```python
from build123d import *

# Parameters (mm, degrees)
BASE_FLANGE1_DEPTH = 631.825
SKETCH2_W          = 25.4
SKETCH2_H          = 6.35
CUT_EXTRUDE1_DEPTH = 50.8
SKETCH3_R          = 3.429
CUT_EXTRUDE2_DEPTH = 3.175
FILLET1_R          = 3.175
SKETCH4_R          = 7.9375
CUT_EXTRUDE3_DEPTH = 3.175


# Sheet-metal steps are written as plain solids
with BuildPart() as part:
    # Sketch1 → Base-Flange1 (new body)
    with BuildSketch(Plane(origin=(0, 0, 0), x_dir=(0, 0, -1), z_dir=(1, 0, 0))):
        with BuildLine():
            Line((31.75, 50.8), (6.35, 50.8))
            ThreePointArc((6.35, 50.8), (1.859871939, 48.940128061), (0, 44.45))
            Line((0, 44.45), (0, 6.35))
            ThreePointArc((0, 6.35), (1.859871939, 1.859871939), (6.35, 0))
            Line((6.35, 0), (31.75, 0))
            Line((31.75, 0), (31.75, 3.175))
            Line((31.75, 3.175), (6.35, 3.175))
            ThreePointArc((6.35, 3.175), (4.10493597, 4.10493597), (3.175, 6.35))
            Line((3.175, 6.35), (3.175, 44.45))
            ThreePointArc((3.175, 44.45), (4.10493597, 46.69506403), (6.35, 47.625))
            Line((6.35, 47.625), (31.75, 47.625))
            Line((31.75, 47.625), (31.75, 50.8))
        make_face()
    extrude(amount=BASE_FLANGE1_DEPTH)

    # Sketch2 → Cut-Extrude1 (cut)
    with BuildSketch(Plane(origin=(0, 50.8, 0), x_dir=(1, 0, 0), z_dir=(0, 1, 0))):
        with Locations((12.7, 28.575)):
            Rectangle(SKETCH2_W, SKETCH2_H)
        with Locations((619.125, 28.575)):
            Rectangle(SKETCH2_W, SKETCH2_H)
    extrude(amount=-CUT_EXTRUDE1_DEPTH, mode=Mode.SUBTRACT)

    # Sketch3 → Cut-Extrude2 (cut)
    with BuildSketch(Plane.XY):
        with Locations((22.225, 19.05)):
            Circle(SKETCH3_R)
        with Locations((22.225, 38.1)):
            Circle(SKETCH3_R)
        with Locations((622.3, 38.1)):
            Circle(SKETCH3_R)
        with BuildLine():
            Line((618.871, 22.225), (618.871, 19.05))
            ThreePointArc((618.871, 19.05), (622.3, 15.621), (625.729, 19.05))
            Line((625.729, 19.05), (625.729, 22.225))
            ThreePointArc((625.729, 22.225), (622.3, 25.654), (618.871, 22.225))
        make_face()
    extrude(amount=-CUT_EXTRUDE2_DEPTH, mode=Mode.SUBTRACT)

    # Fillet1
    fillet1_edges = [part.edges().sort_by_distance(p)[0] for p in [
        (0, 49.2125, -25.4),
        (25.4, 49.2125, -31.75),
        (0, 1.5875, -25.4),
        (25.4, 1.5875, -31.75),
        (606.425, 1.5875, -31.75),
        (606.425, 49.2125, -31.75),
        (631.825, 1.5875, -25.4),
        (631.825, 49.2125, -25.4),
        (606.425, 1.5875, -25.4),
        (606.425, 49.2125, -25.4),
        (25.4, 1.5875, -25.4),
        (25.4, 49.2125, -25.4),
    ]]
    fillet(fillet1_edges, radius=FILLET1_R - 0.0001)  # a hair under: the kernel refuses the full size

    # Sketch4 → Cut-Extrude3 (cut)
    with BuildSketch(Plane.XZ):
        with Locations(Location((41.275, -20.6375, 0), (0, 0, 270))):
            Circle(SKETCH4_R)
    extrude(amount=-CUT_EXTRUDE3_DEPTH, mode=Mode.SUBTRACT)


solid = part.part
```
The listing builds one solid part. Answer for the finished solid, in the listing's coordinates (mm). A direction names the side the tool comes from. Give positions to 0.01 mm unless a question says otherwise; leave off trailing zeros. Write each loop counter-clockwise with the first axis right and the second up, starting at its lowest first coordinate (ties: lowest second). Pieces come first, ordered by that corner, then holes. Notation, with made-up numbers: (-40, 9.5) -> (16, 9.5) arc R29 ccw to (16, 41.5) -> close; hole circle Ø7 at (35.25, 84). An arc over 180 degrees is marked (long way). Write item = value, one per line. Start each with the question number.
1) The part is cut by section A-A, the plane x = 372. Determine the outline of the cut face in (y, z) (3 decimals), and give its area (3 significant figures).
2) Which of the six approach directions +Z, -Z, +X, -X, +Y, -Y give full straight-line access (tool end or side, diameter ignored) to faces 5 (the face through (311, 3.175, -19)), 6 (the face through (311, 0, -19))?
3) Determine the mould class of faces 1 (the face through (631.825, 26, -3)), 2 (the face through (49.145, 1.565, -19.604)), 3 (the face through (311, 26, 0)), 4 (the face through (0, 26, -3)) for opening direction X: +X half, -X half, draft (parallel to the pull), parting line (faces both ways), or undercut.
4) Each of these flat-tipped pins is pushed along its axis until it touches: pin 1 (1.5 mm diameter, centred on x = 252.5, y = 45.5, fed in from +Z); pin 2 (1.6 mm diameter, centred on x = 616, y = 1.5, fed in from -Z); pin 3 (19 mm diameter, centred on x = 357.5, y = 30, fed in from -Z) (3 decimals). Where does it stop, or does it pass through?
5) Straight lines are drawn through the part: line 1 along X through (y, z) = (38, -2) (3 decimals); line 2 along Y through (x, z) = (86.5, -21) (3 decimals); line 3 along Z through (x, y) = (301, 27.5) (3 decimals). For each, find the intervals that lie inside material, in ascending order.
Solutions:
q1.outline = (0, -31.75) -> (3.175, -31.75) -> (3.175, -6.35) arc R3.175 cw to (6.35, -3.175) -> (44.45, -3.175) arc R3.175 cw to (47.625, -6.35) -> (47.625, -31.75) -> (50.8, -31.75) -> (50.8, -6.35) arc R6.35 ccw to (44.45, 0) -> (6.35, 0) arc R6.35 ccw to (0, -6.35) -> close
q1.area = 330 mm²
q2.face_5 = -Z, +X, -X
q2.face_6 = +Z, -Z, +X, -X, -Y
q3.face_1 = +X half
q3.face_2 = undercut
q3.face_3 = draft
q3.face_4 = -X half
q4.pin_1 = -0.01
q4.pin_2 = -25.4
q4.pin_3 = -3.175
q5.line_1 = 0 to 18.797, 25.653 to 618.872, 625.728 to 631.825
q5.line_2 = 0 to 3.175, 47.625 to 50.8
q5.line_3 = -3.175 to 0
